```python
from build123d import *

# Parameters (mm, degrees)
SKETCH2_W               = 57.15
SKETCH2_H               = 41.275
BOSS_EXTRUDE1_DEPTH     = 3.175
SKETCH7_W               = 25.4
SKETCH7_H               = 3.175
BOSS_EXTRUDE2_DEPTH     = 57.15
CUT_EXTRUDE3_DEPTH      = 66.857337528
CUT_EXTRUDE3_DEPTH_BACK = 57.15
FILLET1_R               = 4.953
FILLET2_R               = 6.35
FILLET3_R               = 6.35
SKETCH13_R              = 3.175
CUT_EXTRUDE5_DEPTH      = 57.15
SKETCH14_R              = 3.9751
CUT_EXTRUDE6_DEPTH      = 57.15
CUT_EXTRUDE8_DEPTH      = 42.669985076


with BuildPart() as part:
    # Sketch2 → Boss-Extrude1 (new body)
    with BuildSketch(Plane.XY):
        Rectangle(SKETCH2_W, SKETCH2_H)
    extrude(amount=BOSS_EXTRUDE1_DEPTH)

    # Sketch7 → Boss-Extrude2 (add)
    with BuildSketch(Plane(origin=(28.575, 0, 0), x_dir=(0, 0, -1), z_dir=(1, 0, 0))):
        with Locations((-12.7, -19.05)):
            Rectangle(SKETCH7_W, SKETCH7_H)
    extrude(amount=-BOSS_EXTRUDE2_DEPTH)

    # Sketch8 → Cut-Extrude3 (cut, two sides: drawn at the far end of the back side and taken through both)
    with BuildSketch(Plane(origin=(28.575, 0, 0), x_dir=(0, 0, -1), z_dir=(1, 0, 0)).offset(-CUT_EXTRUDE3_DEPTH_BACK)):
        with BuildLine():
            Line((0, 86.439447679), (0, -15.6845))
            ThreePointArc((0, -15.6845), (-1.450700113, -19.186799887), (-4.953, -20.6375))
            Line((-4.953, -20.6375), (-107.076947679, -20.6375))
            Line((-107.076947679, -20.6375), (37.348124172, -165.062571851))
            Line((37.348124172, -165.062571851), (144.425071851, -57.985624172))
            Line((144.425071851, -57.985624172), (0, 86.439447679))
        make_face()
    extrude(amount=CUT_EXTRUDE3_DEPTH + CUT_EXTRUDE3_DEPTH_BACK, mode=Mode.SUBTRACT)

    # Fillet1
    fillet1_edges = [part.edges().sort_by_distance(p)[0] for p in [
        (0, -17.4625, 3.175),
    ]]
    fillet(fillet1_edges, radius=FILLET1_R)

    # Fillet2
    fillet2_edges = [part.edges().sort_by_distance(p)[0] for p in [
        (28.575, -19.05, 25.4),
    ]]
    fillet(fillet2_edges, radius=FILLET2_R)

    # Fillet3
    fillet3_edges = [part.edges().sort_by_distance(p)[0] for p in [
        (-28.575, -19.05, 25.4),
    ]]
    fillet(fillet3_edges, radius=FILLET3_R)

    # Sketch13 → Cut-Extrude5 (cut)
    with BuildSketch(Plane.XY.offset(3.175)):
        with Locations((-22.350267212, 12.7)):
            Circle(SKETCH13_R)
        with Locations((22.099732788, 12.7)):
            Circle(SKETCH13_R)
    extrude(amount=-CUT_EXTRUDE5_DEPTH, mode=Mode.SUBTRACT)

    # Sketch14 → Cut-Extrude6 (cut)
    with BuildSketch(Plane(origin=(0, -17.4625, 0), x_dir=(1, 0, 0), z_dir=(0, 1, 0))):
        with Locations(Location((-19.05, -15.875, 0), (0, 0, 270))):
            Circle(SKETCH14_R)
        with Locations(Location((19.05, -15.875, 0), (0, 0, 270))):
            Circle(SKETCH14_R)
    extrude(amount=-CUT_EXTRUDE6_DEPTH, mode=Mode.SUBTRACT)

    # Sketch15 → Cut-Extrude8 (cut, through all)
    with BuildSketch(Plane.XY.offset(3.175)):
        with BuildLine():
            ThreePointArc((-22.225, 20.6375), (-20.067470257, 20.259732866), (-18.166647231, 19.171378869))
            Line((-18.166647231, 19.171378869), (-4.058352769, 7.447821131))
            ThreePointArc((-4.058352769, 7.447821131), (0, 5.9817), (4.058352769, 7.447821131))
            Line((4.058352769, 7.447821131), (18.166647231, 19.171378869))
            ThreePointArc((18.166647231, 19.171378869), (20.067470257, 20.259732866), (22.225, 20.6375))
            Line((22.225, 20.6375), (-22.225, 20.6375))
        make_face()
        with BuildLine():
            ThreePointArc((-28.575, 14.2875), (-26.715128061, 18.777628061), (-22.225, 20.6375))
            Line((-22.225, 20.6375), (-28.575, 20.6375))
            Line((-28.575, 20.6375), (-28.575, 14.2875))
        make_face()
        with BuildLine():
            Line((28.575, 20.6375), (22.225, 20.6375))
            ThreePointArc((22.225, 20.6375), (26.715128061, 18.777628061), (28.575, 14.2875))
            Line((28.575, 14.2875), (28.575, 20.6375))
        make_face()
    extrude(amount=-CUT_EXTRUDE8_DEPTH, mode=Mode.SUBTRACT)


solid = part.part
```
Model file for the job. Use its own axes, mm. A direction names the side the tool comes from. Coordinates: 2 decimals unless noted, no trailing zeros. Loops run counter-clockwise (first coordinate to the right, second up) from the corner with the lowest first, then second, coordinate; pieces in that order, holes last. Notation, with made-up numbers: (81, -24) -> (96, -24) arc R17 ccw to (96, -17) -> close; hole circle Ø1 at (-23.5, 49). An arc over 180 degrees is marked (long way). Answer as a JSON object with one key per item and string values.
Q1. Cut at B-B (y = 12.7). List the corners of the cut face in (x, z) (3 decimals), and give its area (3 significant figures).
Report:
{"outline": "(-28.575, 0) -> (-25.525, 0) -> (-25.525, 3.175) -> (-28.575, 3.175) -> close; (-19.175, 0) -> (-10.379, 0) -> (-10.379, 3.175) -> (-19.175, 3.175) -> close; (10.379, 0) -> (18.925, 0) -> (18.925, 3.175) -> (10.379, 3.175) -> close; (25.275, 0) -> (28.575, 0) -> (28.575, 3.175) -> (25.275, 3.175) -> close", "area": "75.2 mm2"}
Q2. Pull direction Z, two halves, no side cores. Call faces 1 (the flat face through (0, 1, 3.175)), 2 (the flat face through (11.014, 13.228, 1.61)), 3 (the cylindrical face through (-21.47, -19.03, 12.72)): released by +Z, released by -Z, zero draft, split by the parting line, or undercut.
Report:
{"face 1": "released by +Z", "face 2": "zero draft", "face 3": "undercut"}
Q3. 3-axis set-ups, long thin cutter, end or side, ignore diameter. For faces 4 (the flat face through (-11.21, 13.39, 1.61)), 5 (the cylindrical face through (26.764, -19.028, 23.49)), 6 (the flat face through (0, -17.463, 17)): which of +Z, -Z, +X, -X, +Y, -Y reach the whole face in a straight line?
Report:
{"face 4": "+Z, -Z, +Y", "face 5": "+Z, +X, +Y, -Y", "face 6": "+Z, +X, -X, +Y"}
Q4. Cut at D-D (x = 13.5). List the corners of the cut face in (y, z) (1 decimal), and give its area (3 significant figures).
Report:
{"outline": "(-20.6, 5) arc R5 ccw to (-15.7, 0) -> (15.3, 0) -> (15.3, 3.2) -> (-12.5, 3.2) arc R5 cw to (-17.5, 8.1) -> (-17.5, 25.4) -> (-20.6, 25.4) -> close", "area": "185 mm2"}
Q5. Flat gauge pins, fed straight in: P1, Ø14, axis at x = 12.5, z = 14, coming from the +Y side; P2, Ø16.5, axis at x = -0.5, y = 10.5, coming from the +Z side (3 decimals); P3, Ø1.5, axis at x = -16, z = 12.5, coming from the +Y side. Where does each tip first touch, or does it go through?
Report:
{"P1": "stops at y = -17.33", "P2": "stops at z = 3.175", "P3": "stops at y = -17.46"}
Q6. Cut at A-A (x = -24). List the corners of the cut face in (y, z) (1 decimal), and give its area (3 significant figures).
Report:
{"outline": "(-20.6, 5) arc R5 ccw to (-15.7, 0) -> (10, 0) -> (10, 3.2) -> (-12.5, 3.2) arc R5 cw to (-17.5, 8.1) -> (-17.5, 25.1) -> (-20.6, 25.1) -> close; (15.4, 0) -> (20.4, 0) -> (20.4, 3.2) -> (15.4, 3.2) -> close", "area": "183 mm2"}
Q7. Probe probe 1 along Y at (x, z) = (24, 19); probe 2 along Z at (x, y) = (13, 12) (3 decimals); probe 3 along Z at (x, y) = (-19, -19). List the from-to ranges inside material, lowest first.
Report:
{"probe 1": "y = -20.64 to -17.46", "probe 2": "z = 0 to 3.175", "probe 3": "z = 1.27 to 11.9, 19.85 to 25.4"}
Q8. Cut at C-C (z = 10.75). List the corners of the cut face in (x, y) (1 decimal).
Report:
{"outline": "(-28.6, -20.6) -> (28.6, -20.6) -> (28.6, -17.5) -> (-28.6, -17.5) -> close"}
